```python
from build123d import *

# Parameters (mm, degrees)
BOSS_EXTRUDE1_DEPTH = 10
BOSS_EXTRUDE2_DEPTH = 10
BOSS_EXTRUDE3_DEPTH = 2


with BuildPart() as part:
    # Sketch1 → Boss-Extrude1 (new body)
    with BuildSketch(Plane.XZ.offset(-112.992351319)):
        with BuildLine():
            Line((-38.224542698, 418.012407464), (30.875674984, 412.996441329))
            ThreePointArc((30.875674984, 412.996441329), (35.013440502, 410.189504116), (34.651444327, 405.202625456))
            Line((34.651444327, 405.202625456), (-4.242618611, 347.868064603))
            ThreePointArc((-4.242618611, 347.868064603), (-8.742380303, 345.688123157), (-12.880145821, 348.49506037))
            Line((-12.880145821, 348.49506037), (-43.086300565, 410.845587357))
            ThreePointArc((-43.086300565, 410.845587357), (-42.724304391, 415.832466017), (-38.224542698, 418.012407464))
        make_face()
    extrude(amount=BOSS_EXTRUDE1_DEPTH)



with BuildPart() as body_2:
    # Sketch3 → Boss-Extrude2 (new body)
    with BuildSketch(Plane.XZ.offset(-102.992351319)):
        with BuildLine():
            Line((-37.500550349, 427.986164784), (31.599667334, 422.970198649))
            ThreePointArc((31.599667334, 422.970198649), (44.012963887, 414.549387009), (42.926975363, 399.588751029))
            Line((42.926975363, 399.588751029), (4.032912425, 342.254190176))
            ThreePointArc((4.032912425, 342.254190176), (-9.466372653, 335.714365837), (-21.879669206, 344.135177477))
            Line((-21.879669206, 344.135177477), (-52.08582395, 406.485704464))
            ThreePointArc((-52.08582395, 406.485704464), (-49.24607828, 420.256643692), (-37.500550349, 427.986164784))
        make_face()
        with BuildLine():
            ThreePointArc((-38.224542698, 418.012407464), (-42.724304391, 415.832466017), (-43.086300565, 410.845587357))
            Line((-43.086300565, 410.845587357), (-12.880145821, 348.49506037))
            ThreePointArc((-12.880145821, 348.49506037), (-8.742380303, 345.688123157), (-4.242618611, 347.868064603))
            Line((-4.242618611, 347.868064603), (34.651444327, 405.202625456))
            ThreePointArc((34.651444327, 405.202625456), (35.013440502, 410.189504116), (30.875674984, 412.996441329))
            Line((30.875674984, 412.996441329), (-38.224542698, 418.012407464))
        make_face(mode=Mode.SUBTRACT)
    extrude(amount=-BOSS_EXTRUDE2_DEPTH)


with BuildPart() as part_1:
    add(part.part)

    add(body_2.part)  # Boss-Extrude3 merges body 2
    # Sketch3_3 → Boss-Extrude3 (add)
    # profile 1 of 2: a face of its own
    with BuildSketch(Plane.XZ.offset(-102.992351319)):
        with BuildLine():
            Line((-37.500550349, 427.986164784), (31.599667334, 422.970198649))
            ThreePointArc((31.599667334, 422.970198649), (44.012963887, 414.549387009), (42.926975363, 399.588751029))
            Line((42.926975363, 399.588751029), (4.032912425, 342.254190176))
            ThreePointArc((4.032912425, 342.254190176), (-9.466372653, 335.714365837), (-21.879669206, 344.135177477))
            Line((-21.879669206, 344.135177477), (-52.08582395, 406.485704464))
            ThreePointArc((-52.08582395, 406.485704464), (-49.24607828, 420.256643692), (-37.500550349, 427.986164784))
        make_face()
        with BuildLine():
            ThreePointArc((-38.224542698, 418.012407464), (-42.724304391, 415.832466017), (-43.086300565, 410.845587357))
            Line((-43.086300565, 410.845587357), (-12.880145821, 348.49506037))
            ThreePointArc((-12.880145821, 348.49506037), (-8.742380303, 345.688123157), (-4.242618611, 347.868064603))
            Line((-4.242618611, 347.868064603), (34.651444327, 405.202625456))
            ThreePointArc((34.651444327, 405.202625456), (35.013440502, 410.189504116), (30.875674984, 412.996441329))
            Line((30.875674984, 412.996441329), (-38.224542698, 418.012407464))
        make_face(mode=Mode.SUBTRACT)
    # profile 2 of 2: a face of its own
    with BuildSketch(Plane.XZ.offset(-102.992351319)):
        with BuildLine():
            Line((30.875674984, 412.996441329), (-38.224542698, 418.012407464))
            ThreePointArc((-38.224542698, 418.012407464), (-42.724304391, 415.832466017), (-43.086300565, 410.845587357))
            Line((-43.086300565, 410.845587357), (-12.880145821, 348.49506037))
            ThreePointArc((-12.880145821, 348.49506037), (-8.742380303, 345.688123157), (-4.242618611, 347.868064603))
            Line((-4.242618611, 347.868064603), (34.651444327, 405.202625456))
            ThreePointArc((34.651444327, 405.202625456), (35.013440502, 410.189504116), (30.875674984, 412.996441329))
        make_face()
    extrude(amount=BOSS_EXTRUDE3_DEPTH)


solid = part_1.part
```
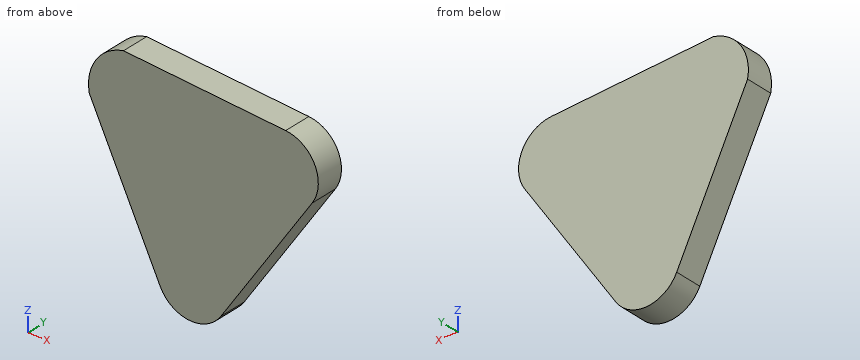
Geometry check sheet. Reference: the model listing, model coordinates, mm. Coordinates: 2 decimals unless noted, no trailing zeros. Loops run counter-clockwise (first coordinate to the right, second up) from the corner with the lowest first, then second, coordinate; pieces in that order, holes last.
Item 1: Sectioned sample at A-A, the plane y = 111.25. Record the boundary of the cut face in (x, z) (3 decimals), then the cut area to 3 significant figures.
Item 2: Sectioned sample at C-C, the plane x = -20.5. Record the boundary of the cut face in (y, z), then the cut area to 3 significant figures.
Item 3: Go/stop test with flat-tipped pins: pin 1 Ø5 at (x, y) = (1, 103.5) entering from -Z; pin 2 Ø2 at (y, z) = (106.5, 393.5) entering from +X; pin 3 Ø1.5 at (y, z) = (110, 406.5) entering from -X; pin 4 Ø1.5 at (x, z) = (-29.5, 354) entering from -Y. Record where each tip stops, or that it passes through.
Item 4: Sectioned sample at B-B, the plane z = 366. Record the boundary of the cut face in (x, y).
Item 5: Thickness scan on line 1 (Z direction, x = 17.5, y = 105.5); line 2 (Z direction, x = 1.5, y = 103.25); line 3 (X direction, y = 106, z = 374). Record the ranges inside material, lowest first.
Check result:
1. outline: (-52.086, 406.486) - (-21.88, 344.135) arc R15 ccw to (4.033, 342.254) - (42.927, 399.589) arc R15 ccw to (31.6, 422.97) - (-37.501, 427.986) arc R18.371 ccw to start
1. area: 5,860 mm2
2. outline: (100.99, 341.84) - (112.99, 341.84) - (112.99, 426.75) - (100.99, 426.75) - close
2. area: 1,020 mm2
3. pin 1: stops at z = 337.35
3. pin 2: stops at x = 39.47
3. pin 3: stops at x = -52.22
3. pin 4: passes through
4. outline: (-32.47, 100.99) - (20.14, 100.99) - (20.14, 112.99) - (-32.47, 112.99) - close
5. line 1: z = 362.11 to 423.99
5. line 2: z = 339.39 to 425.16
5. line 3: x = -36.35 to 25.57
